from build123d import *

# Parameters (mm, degrees)
SKETCH_2_R          = 2
EXTRUDE_1_DEPTH     = 6
SKETCH_3_R          = 2
EXTRUDE_2_DEPTH     = 6
SKETCH_4_R          = 2
EXTRUDE_3_DEPTH     = 6
SKETCH_6_R          = 0.9
CUT_EXTRUDE_1_DEPTH = 5
SKETCH_10_R         = 1.25
EXTRUDE_4_DEPTH     = 5
SKETCH_7_R          = 0.9
CUT_EXTRUDE_2_DEPTH = 5
SKETCH_8_R          = 0.9
CUT_EXTRUDE_3_DEPTH = 5
SKETCH_14_R         = 0.65
CUT_EXTRUDE_4_DEPTH = 3


with BuildPart() as part:
    # 草图2 → 凸台-拉伸1 (new body)
    with BuildSketch(Plane(origin=(0, 0, 0), x_dir=(1, 0, 0), z_dir=(0, 1, 0))):
        with Locations(Location((0, 0, 0), (0, 0, 270))):
            Circle(SKETCH_2_R)
    extrude(amount=EXTRUDE_1_DEPTH)

    # 草图3 → 凸台-拉伸2 (add)
    with BuildSketch(Plane.XY):
        Circle(SKETCH_3_R)
    extrude(amount=EXTRUDE_2_DEPTH)

    # 草图4 → 凸台-拉伸3 (add)
    with BuildSketch(Plane(origin=(0, 0, 0), x_dir=(0, 0, -1), z_dir=(1, 0, 0))):
        Circle(SKETCH_4_R)
    extrude(amount=EXTRUDE_3_DEPTH)

    # 草图5 → 旋转3 (revolve)
    with BuildSketch(Plane(origin=(0, 0, 0), x_dir=(1, 0, 0), z_dir=(0, 1, 0))):
        with BuildLine():
            Line((0, 2.5), (0, -2.5))
            ThreePointArc((0, -2.5), (-2.5, 0), (0, 2.5))
        make_face()
    revolve(axis=Axis((0, 0, -2.5), (0, 0, 1)))

    # 草图6 → 切除-拉伸1 (cut)
    with BuildSketch(Plane(origin=(0, 6, 0), x_dir=(1, 0, 0), z_dir=(0, 1, 0))):
        with Locations(Location((0, 0, 0), (0, 0, 270))):
            Circle(SKETCH_6_R)
    extrude(amount=-CUT_EXTRUDE_1_DEPTH, mode=Mode.SUBTRACT)

    # 草图10 → 凸台-拉伸4 (add)
    with BuildSketch(Plane(origin=(0, 0, 0), x_dir=(0.7071067811865461, 0, -0.707106781186549), z_dir=(0.707106781186549, 0, 0.7071067811865461))):
        with Locations(Location((0, 0, 0), (0, 0, 90.000016419))):
            Circle(SKETCH_10_R)
    extrude(amount=EXTRUDE_4_DEPTH)

    # 草图7 → 切除-拉伸2 (cut)
    with BuildSketch(Plane(origin=(6, 0, 0), x_dir=(0, 0, -1), z_dir=(1, 0, 0))):
        Circle(SKETCH_7_R)
    extrude(amount=-CUT_EXTRUDE_2_DEPTH, mode=Mode.SUBTRACT)

    # 草图8 → 切除-拉伸3 (cut)
    with BuildSketch(Plane.XY.offset(6)):
        Circle(SKETCH_8_R)
    extrude(amount=-CUT_EXTRUDE_3_DEPTH, mode=Mode.SUBTRACT)

    # 草图14 → 切除-拉伸4 (cut)
    with BuildSketch(Plane(origin=(3.535533906, 0, 3.535533906), x_dir=(0.7071067811865462, 0, -0.7071067811865489), z_dir=(0.7071067811865489, 0, 0.7071067811865462))):
        Circle(SKETCH_14_R)
    extrude(amount=-CUT_EXTRUDE_4_DEPTH, mode=Mode.SUBTRACT)


solid = part.part
Read the model definition and answer for the solid it produces. Units are mm, in the model's axes. A direction names the side the tool comes from. Coordinates: 2 decimals unless noted, no trailing zeros. Order: outer loops, then holes, each group sorted by start corner. A loop starts at its lowest first (then second) coordinate and runs counter-clockwise, first axis right, second up. Notation, with made-up numbers: (85, -11) - (122, -11) arc R25 ccw to (122, 5) - close; hole circle Ø6 at (31.5, 66). An arc over 180 degrees is marked (long way). Use one line per item in the form item = value.
(1) Given pin 1 Ø3 at (x, z) = (2, 2) entering from -Y; pin 2 Ø1 at (y, z) = (1.5, 4) entering from -X; pin 3 Ø1.5 at (x, y) = (4.5, 4.5) entering from -Z; pin 4 Ø0.5 at (y, z) = (0.5, 0) entering from +X, each flat-ended and moving along its own axis, determine where each tip first touches the part or whether it passes through.
Computed values:
pin_1 = -2.12
pin_2 = -1.73
pin_3 = through
pin_4 = 1
(2) For a pull along X with two mould halves and no side action, classify faces 5 (the face through (-1.2, 3.7, -1.6)), 6 (the face through (-0.2, 1, -0.2)), 7 (the face through (4.11, -0.02, 2.96)) as pulls with the +X half, pulls with the -X half, needs draft (parallel to the pull), parting line crosses it, or undercut.
Computed values:
face_5 = parting line crosses it
face_6 = undercut
face_7 = pulls with the +X half
(3) Section D-D, the plane x = -0.75 is taken. Give the vertices of the cut face in (y, z).
Computed values:
outline = (-1.85, 1.5) arc R2.38 ccw to (1.5, -1.85) - (6, -1.85) - (6, -0.5) - (1, -0.5) - (1, 0.5) - (6, 0.5) - (6, 1.85) - (1.85, 1.85) - (1.85, 6) - (0.5, 6) - (0.5, 1) - (-0.5, 1) - (-0.5, 6) - (-1.85, 6) - close
(4) Section A-A, the plane y = 0.5 is taken. Give the vertices of the cut face in (x, z).
Computed values:
outline = (-1.94, 1.5) arc R2.45 ccw to (1.5, -1.94) - (6, -1.94) - (6, -0.75) - (1, -0.75) - (1, 0.75) - (6, 0.75) - (6, 1.94) - (3.56, 1.94) - (4.35, 2.73) - (3.83, 3.24) - (1.71, 1.12) - (1.12, 1.71) - (3.24, 3.83) - (2.73, 4.35) - (1.94, 3.56) - (1.94, 6) - (0.75, 6) - (0.75, 1) - (-0.75, 1) - (-0.75, 6) - (-1.94, 6) - close
(5) Which of the six approach directions +Z, -Z, +X, -X, +Y, -Y give full straight-line access (tool end or side, diameter ignored) to faces 1 (the face through (0, 0, 1)), 2 (the face through (3.54, 0.27, -0.86)), 3 (the face through (1.41, 0.01, 1.42)), 4 (the face through (-0.345, 3.535, 0.831))?
Computed values:
face_1 = +Z
face_2 = +X
face_3 = none
face_4 = +Y
(6) A straight line is drawn through the part: L1, parallel to Y at x = 0, z = 2.1. Find the intervals that lie inside material, in ascending order.
Computed values:
L1 = -2 to -0.9, 0.9 to 2
(7) Section B-B, the plane z = 5 is taken. Give the vertices of the cut face in (x, y).
Computed values:
outline = circle Ø4 at (0, 0); hole circle Ø1.8 at (0, 0)
